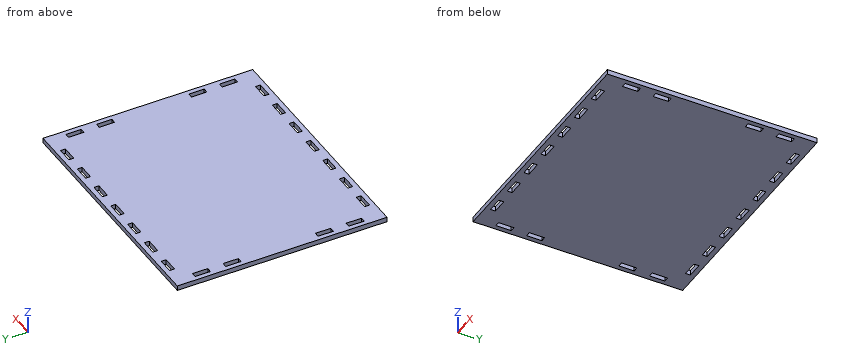
```python
from build123d import *

# Parameters (mm, degrees)
SKETCH1_W           = 160
SKETCH1_H           = 136.35
SKETCH1_W_2         = 10
SKETCH1_H_2         = 3.175
SKETCH1_W_3         = 3.175
SKETCH1_H_3         = 10
BOSS_EXTRUDE1_DEPTH = 3.175


with BuildPart() as part:
    # Sketch1 → Boss-Extrude1 (new body)
    with BuildSketch(Plane.XY):
        with Locations((80, 68.069958461)):
            Rectangle(SKETCH1_W, SKETCH1_H)
        with Locations((40, 131.482458461)):
            Rectangle(SKETCH1_W_2, SKETCH1_H_2, mode=Mode.SUBTRACT)
        with Locations((20, 131.482458461)):
            Rectangle(SKETCH1_W_2, SKETCH1_H_2, mode=Mode.SUBTRACT)
        with Locations((60, 131.482458461)):
            Rectangle(SKETCH1_W_2, SKETCH1_H_2, mode=Mode.SUBTRACT)
        with Locations((80, 131.482458461)):
            Rectangle(SKETCH1_W_2, SKETCH1_H_2, mode=Mode.SUBTRACT)
        with Locations((100, 131.482458461)):
            Rectangle(SKETCH1_W_2, SKETCH1_H_2, mode=Mode.SUBTRACT)
        with Locations((120, 131.482458461)):
            Rectangle(SKETCH1_W_2, SKETCH1_H_2, mode=Mode.SUBTRACT)
        with Locations((140, 131.482458461)):
            Rectangle(SKETCH1_W_2, SKETCH1_H_2, mode=Mode.SUBTRACT)
        with Locations((140, 4.657458461)):
            Rectangle(SKETCH1_W_2, SKETCH1_H_2, mode=Mode.SUBTRACT)
        with Locations((120, 4.657458461)):
            Rectangle(SKETCH1_W_2, SKETCH1_H_2, mode=Mode.SUBTRACT)
        with Locations((100, 4.657458461)):
            Rectangle(SKETCH1_W_2, SKETCH1_H_2, mode=Mode.SUBTRACT)
        with Locations((80, 4.657458461)):
            Rectangle(SKETCH1_W_2, SKETCH1_H_2, mode=Mode.SUBTRACT)
        with Locations((60, 4.657458461)):
            Rectangle(SKETCH1_W_2, SKETCH1_H_2, mode=Mode.SUBTRACT)
        with Locations((40, 4.657458461)):
            Rectangle(SKETCH1_W_2, SKETCH1_H_2, mode=Mode.SUBTRACT)
        with Locations((20, 4.657458461)):
            Rectangle(SKETCH1_W_2, SKETCH1_H_2, mode=Mode.SUBTRACT)
        with Locations((4.5875, 38.069958461)):
            Rectangle(SKETCH1_W_3, SKETCH1_H_3, mode=Mode.SUBTRACT)
        with Locations((4.5875, 98.069958461)):
            Rectangle(SKETCH1_W_3, SKETCH1_H_3, mode=Mode.SUBTRACT)
        with Locations((4.5875, 118.069958461)):
            Rectangle(SKETCH1_W_3, SKETCH1_H_3, mode=Mode.SUBTRACT)
        with Locations((4.5875, 18.069958461)):
            Rectangle(SKETCH1_W_3, SKETCH1_H_3, mode=Mode.SUBTRACT)
        with Locations((155.4125, 18.069958461)):
            Rectangle(SKETCH1_W_3, SKETCH1_H_3, mode=Mode.SUBTRACT)
        with Locations((155.4125, 38.069958461)):
            Rectangle(SKETCH1_W_3, SKETCH1_H_3, mode=Mode.SUBTRACT)
        with Locations((155.4125, 98.069958461)):
            Rectangle(SKETCH1_W_3, SKETCH1_H_3, mode=Mode.SUBTRACT)
        with Locations((155.4125, 118.069958461)):
            Rectangle(SKETCH1_W_3, SKETCH1_H_3, mode=Mode.SUBTRACT)
    extrude(amount=BOSS_EXTRUDE1_DEPTH)


solid = part.part
```
Part model, mm, in its own coordinate system. Coordinates: 2 decimals unless noted, no trailing zeros. Loops run counter-clockwise (first coordinate to the right, second up) from the corner with the lowest first, then second, coordinate; pieces in that order, holes last. Notation, with made-up numbers: (78, 65.25) - (109, 65.25) arc R9 ccw to (109, 77.25) - close; hole circle Ø9 at (77.5, 16.25). An arc over 180 degrees is marked (long way). Write item = value, one per line. Start each with the question number.
Item 1: Cut at A-A, the plane x = 103. Give the cut face in (y, z) (3 decimals), and give its area (3 significant figures).
Item 2: Cut at B-B, the plane z = 1.8. State how many separate pieces and enclosed holes the cut face has, and give its area (3 significant figures).
Item 3: Wall check: L1, parallel to X at y = 96.5, z = 2.6 (3 decimals); L2, parallel to Y at x = 140, z = 2.25. Give the ranges that are in metal, low to high. Write a range as from..to.
The answers:
q1.outline = (-0.105, 0) - (3.07, 0) - (3.07, 3.175) - (-0.105, 3.175) - close; (6.245, 0) - (129.895, 0) - (129.895, 3.175) - (6.245, 3.175) - close; (133.07, 0) - (136.245, 0) - (136.245, 3.175) - (133.07, 3.175) - close
q1.area = 413 mm2
q2.separate_pieces = 1
q2.enclosed_holes = 22
q2.area = 21,100 mm2
q3.L1 = 0..3, 6.175..153.825, 157..160
q3.L2 = -0.11..3.07, 6.24..129.89, 133.07..136.24
